```python
from build123d import *

# Parameters (mm, degrees)
SKETCH1_W           = 290
SKETCH1_H           = 30
BOSS_EXTRUDE1_DEPTH = 50
CUT_EXTRUDE3_REACH  = 32
SKETCH5_R           = 12.5
SKETCH7_W           = 194
SKETCH7_H           = 100
SKETCH7_R           = 12.5
BOSS_EXTRUDE2_DEPTH = 25
FILLET1_R           = 30
SKETCH8_R           = 12.5
BOSS_EXTRUDE3_DEPTH = 25
SKETCH9_R           = 50
SKETCH9_R_2         = 30
BOSS_EXTRUDE4_DEPTH = 56


with BuildPart() as part:
    # Sketch1 → Boss-Extrude1 (new body, symmetric)
    with BuildSketch(Plane.XY):
        with Locations((145, 15)):
            Rectangle(SKETCH1_W, SKETCH1_H)
    extrude(amount=BOSS_EXTRUDE1_DEPTH, both=True)

    # Sketch5 → Cut-Extrude3 (cut, up to next)
    with BuildSketch(Plane(origin=(0, 0, 0), x_dir=(1, 0, 0), z_dir=(0, 1, 0)), mode=Mode.PRIVATE) as cut_extrude3_sk1:
        with Locations(Location((36, 0, 0), (0, 0, 90))):  # turned: the seam where the file's is
            Circle(SKETCH5_R)
    cut_extrude3_tool1 = extrude(cut_extrude3_sk1.sketch, amount=CUT_EXTRUDE3_REACH, mode=Mode.PRIVATE) & part.part
    add(cut_extrude3_tool1.solids().sort_by_distance((36, 0, 0))[0], mode=Mode.SUBTRACT)
    # Sketch5 → Cut-Extrude3 (cut, up to next)
    with BuildSketch(Plane(origin=(0, 0, 0), x_dir=(1, 0, 0), z_dir=(0, 1, 0)), mode=Mode.PRIVATE) as cut_extrude3_sk2:
        with Locations(Location((254, 0, 0), (0, 0, 90))):  # turned: the seam where the file's is
            Circle(SKETCH5_R)
    cut_extrude3_tool2 = extrude(cut_extrude3_sk2.sketch, amount=CUT_EXTRUDE3_REACH, mode=Mode.PRIVATE) & part.part
    add(cut_extrude3_tool2.solids().sort_by_distance((254, 0, 0))[0], mode=Mode.SUBTRACT)

    # Sketch7 → Boss-Extrude2 (add)
    with BuildSketch(Plane.XY.offset(50)):
        with Locations((157, 80)):
            Rectangle(SKETCH7_W, SKETCH7_H)
        with Locations((90, 100)):
            Circle(SKETCH7_R, mode=Mode.SUBTRACT)
    extrude(amount=-BOSS_EXTRUDE2_DEPTH)

    # Fillet1
    fillet1_edges = [part.edges().sort_by_distance(p)[0] for p in [
        (254, 130, 37.5),
        (60, 130, 37.5),
    ]]
    fillet(fillet1_edges, radius=FILLET1_R)

    # Sketch8 → Boss-Extrude3 (add)
    with BuildSketch(Plane(origin=(0, 0, -50), x_dir=(-1, 0, 0), z_dir=(0, 0, -1))):
        with BuildLine():
            Line((-90, 130), (-224, 130))
            ThreePointArc((-224, 130), (-245.213203436, 121.213203436), (-254, 100))
            Line((-254, 100), (-254, 30))
            Line((-254, 30), (-60, 30))
            Line((-60, 30), (-60, 100))
            ThreePointArc((-60, 100), (-68.786796564, 121.213203436), (-90, 130))
        make_face()
        with Locations(Location((-90, 100, 0), (0, 0, 180))):  # turned: the seam where the file's is
            Circle(SKETCH8_R, mode=Mode.SUBTRACT)
    extrude(amount=-BOSS_EXTRUDE3_DEPTH)

    # Sketch9 → Boss-Extrude4 (add, symmetric)
    with BuildSketch(Plane.XY):
        with Locations((180, 100)):
            Circle(SKETCH9_R)
        with Locations(Location((180, 100, 0), (0, 0, 180))):  # turned: the seam where the file's is
            Circle(SKETCH9_R_2, mode=Mode.SUBTRACT)
    extrude(amount=BOSS_EXTRUDE4_DEPTH, both=True)


solid = part.part
```
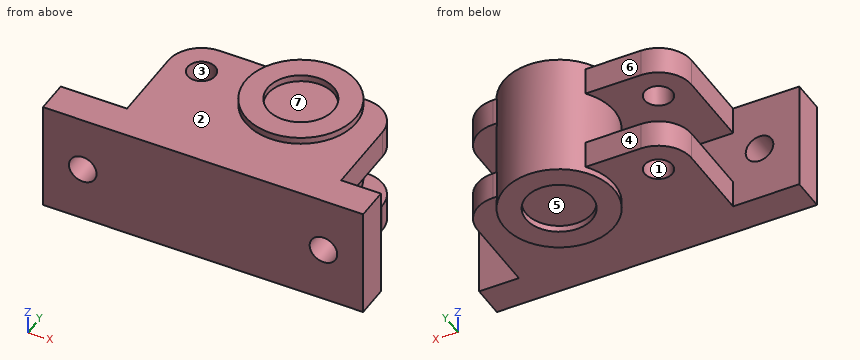
The listing builds one solid part. Answer for the finished solid, in the listing's coordinates (mm). Face numbers are marked on the shaded views. A direction names the side the tool comes from. Coordinates: 2 decimals unless noted, no trailing zeros. Write each loop counter-clockwise with the first axis right and the second up, starting at its lowest first coordinate (ties: lowest second). Pieces come first, ordered by that corner, then holes. Notation, with made-up numbers: (61, 37.5) - (116, 37.5) arc R30 ccw to (116, 63.5) - close; hole circle Ø11 at (10.25, 77.5). An arc over 180 degrees is marked (long way). Return JSON: item names as keys, results as strings. Group by question number.
Q1. Flat-ended cylindrical pins translate along their axes: pin 1 Ø5 at (x, y) = (220, 54.5) entering from -Z; pin 2 Ø4.5 at (x, z) = (221, 31.5) entering from +Y; pin 3 Ø12 at (x, z) = (41, -33) entering from +Y; pin 4 Ø6 at (x, z) = (121, 11.5) entering from -Y. Find the tip coordinate at first contact, or state that the pin passes through.
Q2. For a pull along Y with two mould halves and no side action, classify the marked faces 1, 2, 3 and 4 as +Y half, -Y half, draft (parallel to the pull), parting line (faces both ways), or undercut.
Q3. The part is cut by section C-C on z = 28. Write down the section's boundary in (x, y), and give its area (3 significant figures).
Q4. Which of the six approach directions +Z, -Z, +X, -X, +Y, -Y give full straight-line access (tool end or side, diameter ignored) to the marked faces 5, 6 and 7?
Q5. The part is cut by section A-A on z = 0. Write down the section's boundary in (x, y), and give its area (3 significant figures).
Q6. Find the intervals of material crossed by line 1 along X through (y, z) = (23, 0); line 2 along Y through (x, z) = (182, -3); line 3 along X through (y, z) = (100, -2), in increasing order. Write a range as [from, to].
Q7. The part is cut by section B-B on x = 36. Write down the section's boundary in (y, z), and give its area (3 significant figures).
Evaluation:
{
 "1": {"pin 1": "stops at z = -50", "pin 2": "stops at y = 131.6", "pin 3": "stops at y = 30", "pin 4": "stops at y = 0"},
 "2": {"face 1": "undercut", "face 2": "draft", "face 3": "undercut", "face 4": "+Y half"},
 "3": {"outline": "(0, 0) - (290, 0) - (290, 30) - (254, 30) - (254, 100) arc R30 ccw to (224, 130) - (220, 130) arc R50 ccw to (140, 130) - (90, 130) arc R30 ccw to (60, 100) - (60, 30) - (0, 30) - close; hole circle Ø25 at (90, 100)", "area": "28,300 mm2"},
 "4": {"face 5": "-Z", "face 6": "+Z, -Z, -X, +Y", "face 7": "+Z"},
 "5": {"outline": "(0, 0) - (23.5, 0) - (23.5, 30) - (0, 30) - close; (48.5, 0) - (241.5, 0) - (241.5, 30) - (48.5, 30) - close; circle Ø100 at (180, 100); (266.5, 0) - (290, 0) - (290, 30) - (266.5, 30) - close; hole circle Ø60 at (180, 100)", "area": "12,200 mm2"},
 "6": {"line 1": "x = [0, 23.5], [48.5, 241.5], [266.5, 290]", "line 2": "y = [0, 30], [50.04, 70.07], [129.93, 149.96]", "line 3": "x = [130, 150], [210, 230]"},
 "7": {"outline": "(0, -50) - (30, -50) - (30, -12.5) - (0, -12.5) - close; (0, 12.5) - (30, 12.5) - (30, 50) - (0, 50) - close", "area": "2,250 mm2"}
}
